```python
from build123d import *


with BuildPart() as f1:
    # F0 (on Top) → F1 (revolve)
    with BuildSketch(Plane.XY):
        with BuildLine():
            Line((-115.5733242631, 57.0293739438), (-115.5733242631, -75.9797766805))
            Line((-115.5733242631, -75.9797766805), (-49.7417673469, -69.1965743899))
            Line((-49.7417673469, -69.1965743899), (-53.5328015685, 68.2412087917))
            add(Edge.make_bspline(
                [(-61.6601034999, 74.4477882981), (-60.1760774382, 74.783803467), (-56.7265722306, 75.5648450568), (-54.6920458476, 70.8994721239), (-53.5328015685, 68.2412087917)],
                knots=[0, 0, 0, 0, 0.4302141822, 1, 1, 1, 1], degree=3))
            Line((-61.6601034999, 74.4477882981), (-61.6601034999, 82.4199629432))
            Line((-61.6601034999, 82.4199629432), (-108.8746339083, 77.5962844491))
            Line((-108.8746339083, 77.5962844491), (-108.8746339083, 67.8164288402))
            add(Edge.make_bspline(
                [(-115.5733242631, 57.0293739438), (-114.8918775977, 61.1384455934), (-113.7933541673, 67.7624584675), (-110.2282124707, 67.8015767779), (-108.8746339083, 67.8164288402)],
                knots=[0, 0, 0, 0, 0.6203296593, 1, 1, 1, 1], degree=3))
        make_face()
    revolve(axis=Axis((-115.5733242631, -9.4752013683, 0), (0, 1, 0)))


solid = f1.part
```
CAD build for the part. Positions are in the model's coordinates, mm. Give positions to 0.01 mm unless a question says otherwise; leave off trailing zeros. Order: outer loops, then holes, each group sorted by start corner. A loop starts at its lowest first (then second) coordinate and runs counter-clockwise, first axis right, second up. Notation, with made-up numbers: M -30.75,21.5 L 9.25,21.5 A16 ccw 9.25,32.5 Z; hole C 0.25,0.25 d2. An arc over 180 degrees is marked long. Put each result on its own line as item: value. Start each with the question number.
(1) Mould opens along Z. For faces 1 (the conical face through (-111.645, -75.555, -1.237)), 2 (the cylindrical face through (-122.266, 72.638, -0.295)) say: +Z half, -Z half, draft (parallel to the pull), parting line (faces both ways), or undercut.
(2) Drill centre lines: line 1 along X through (y, z) = (75.25, 0); line 2 along X through (y, z) = (72.5, 0); line 3 along X through (y, z) = (19, 29.5). Where is each one in solid material? Low to high.
(3) Flat gauge pins, fed straight in: pin 1 Ø10 at (x, z) = (-148, 5) entering from +Y; pin 2 Ø3 at (y, z) = (54, 32) entering from -X; pin 3 Ø4 at (x, z) = (-95, 19.5) entering from -Y. Where does each tip first touch, or does it go through?
(4) Saw through at B-B, the plane y = 11. Write the cut outline in (x, z), then the cut area to 3 significant figures.
(5) Saw through at A-A, the plane y = 49.5. Write the cut outline in (x, z).
Check result:
1. face 1: parting line
1. face 2: undercut
2. line 1: x = -169.49 to -122.27, -108.87 to -61.66
2. line 2: x = -175.52 to -122.27, -108.87 to -55.63
2. line 3: x = -171.69 to -59.46
3. pin 1: stops at y = 80.77
3. pin 2: stops at x = -170.05
3. pin 3: stops at y = -73.27
4. outline: C -115.57,0 d127.24
4. area: 12,700 mm2
5. outline: C -115.57,0 d125.11
